from build123d import *

# Parameters (mm, degrees)
SKETCH1_W           = 339.05
SKETCH1_H           = 123
BOSS_EXTRUDE1_DEPTH = 3.175
SKETCH2_W           = 3.175
SKETCH2_H           = 30
CUT_EXTRUDE1_DEPTH  = 10
SKETCH3_W           = 40
SKETCH3_H           = 3.175
CUT_EXTRUDE2_DEPTH  = 361.685435144
LPATTERN1_COUNT     = 3
LPATTERN1_PITCH     = 106.35


with BuildPart() as part:
    # Sketch1 → Boss-Extrude1 (new body)
    with BuildSketch(Plane(origin=(0, 0, 0), x_dir=(0, 0, -1), z_dir=(1, 0, 0))):
        with Locations((169.525, -61.5)):
            Rectangle(SKETCH1_W, SKETCH1_H)
    extrude(amount=BOSS_EXTRUDE1_DEPTH)

    # Sketch2 → Cut-Extrude1 (cut)
    with BuildSketch(Plane(origin=(3.175, 0, 0), x_dir=(0, 0, -1), z_dir=(1, 0, 0))):
        with Locations((337.4625, -35)):
            Rectangle(SKETCH2_W, SKETCH2_H)
        with Locations((337.4625, -95)):
            Rectangle(SKETCH2_W, SKETCH2_H)
        with Locations((1.5875, -35)):
            Rectangle(SKETCH2_W, SKETCH2_H)
        with Locations((1.5875, -95)):
            Rectangle(SKETCH2_W, SKETCH2_H)
    extrude(amount=-CUT_EXTRUDE1_DEPTH, mode=Mode.SUBTRACT)

    # Sketch3 → Cut-Extrude2 (cut, through all)
    with BuildSketch(Plane(origin=(3.175, 0, 0), x_dir=(0, 0, -1), z_dir=(1, 0, 0))):
        with Locations((63.18, -121.4125)):
            Rectangle(SKETCH3_W, SKETCH3_H)
    cut_extrude2 = extrude(amount=-CUT_EXTRUDE2_DEPTH, mode=Mode.SUBTRACT)

    # LPattern1: Cut-Extrude2 ×3
    with Locations(*[(0, 0, -i * LPATTERN1_PITCH) for i in range(1, LPATTERN1_COUNT)]):
        add(cut_extrude2, mode=Mode.SUBTRACT)


solid = part.part
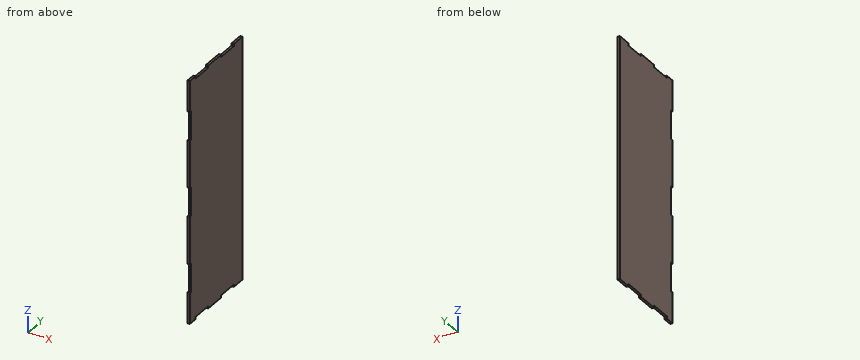
Build history of the part. All positions in model axes, mm. Coordinates: 2 decimals unless noted, no trailing zeros. Order: outer loops, then holes, each group sorted by start corner. A loop starts at its lowest first (then second) coordinate and runs counter-clockwise, first axis right, second up. Notation, with made-up numbers: (27, 30.25) - (41, 30.25) arc R19 ccw to (41, 61.25) - close; hole circle Ø6 at (40.25, -37.75). An arc over 180 degrees is marked (long way). Write item = value, one per line. Start each with the question number.
1) Saw through at C-C on y = -96. Write the cut outline in (x, z) (3 decimals).
2) Wall check: line 1 along Z through (x, y) = (2.35, -104.5) (3 decimals); line 2 along Y through (x, z) = (0.15, -153.5) (3 decimals). Give the ranges that are in metal, low to high. Write a range as from..to.
3) Flat gauge pins, fed straight in: pin 1 Ø1 at (x, z) = (1.5, -61) entering from -Y (3 decimals); pin 2 Ø1.5 at (x, y) = (3, -85.5) entering from +Z (3 decimals). Where does each tip first touch, or does it go through?
4) Saw through at B-B on z = -54. Write the cut outline in (x, y) (3 decimals), then the cut area to 3 significant figures.
From the geometry:
q1.outline = (0, -335.875) - (3.175, -335.875) - (3.175, -3.175) - (0, -3.175) - close
q2.line_1 = -335.875..-3.175
q2.line_2 = -119.825..0
q3.pin_1 = -119.825
q3.pin_2 = -3.175
q4.outline = (0, -119.825) - (3.175, -119.825) - (3.175, 0) - (0, 0) - close
q4.area = 380 mm^2
